Input: part model. Units: mm. Frame: model coordinates. Face numbers are marked on the shaded views. A direction names the side the tool comes from. Coordinates: 2 decimals unless noted, no trailing zeros. Loops run counter-clockwise (first coordinate to the right, second up) from the corner with the lowest first, then second, coordinate; pieces in that order, holes last. Notation, with made-up numbers: M 75,68 L 100,68 A28 cw 100,86 Z; hole C 30,-14 d11. An arc over 180 degrees is marked long. Use a Markdown table: item, result. Add a question column.
1. Section A-A on z = 0. Output: boundary loops of the cut face in (x, y), then the cut area to 3 significant figures.
2. Line query: L1, parallel to Y at x = 18, z = 18; L2, parallel to Y at x = 2.5, z = 13.5; L3, parallel to Z at x = 21, y = 36.5. Output: solid intervals per line, ascending. Write a range as [from, to].
3. Section C-C on x = 28. Output: boundary loops of the cut face in (y, z), then the cut area to 3 significant figures.
4. Pin query (flat end, axial travel): pin 1 (6 mm diameter, centred on x = 14.5, z = -2.5, fed in from +Y); pin 2 (3 mm diameter, centred on x = 17, z = 27.5, fed in from -Y); pin 3 (1.5 mm diameter, centred on x = 22, y = 1.5, fed in from -Z). Return the tip coordinate at first contact, or that it passes through.
5. Set-up query: the marked faces 1 and 2. Return all of +Z, -Z, +X, -X, +Y, -Y with unobstructed straight access to the full face (end or side cutting, diameter ignored); none if empty.
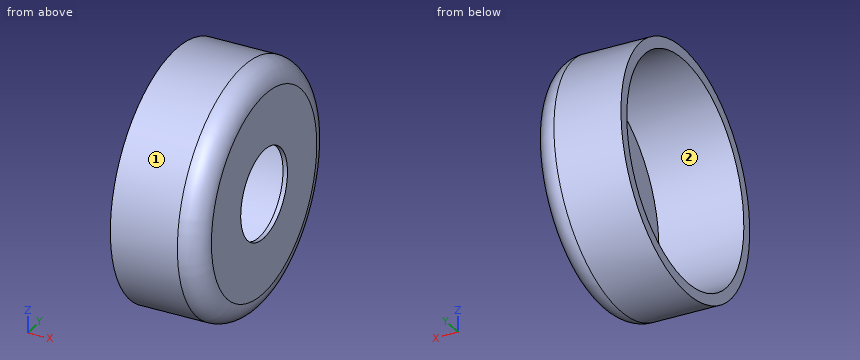
```python
from build123d import *

# Parameters (mm, degrees)
SKETCH1_R           = 55
BOSS_EXTRUDE1_DEPTH = 40
SKETCH2_R           = 50
CUT_EXTRUDE1_DEPTH  = 38
SKETCH3_R           = 20
CUT_EXTRUDE2_DEPTH  = 38
FILLET1_R           = 10


with BuildPart() as part:
    # Sketch1 → Boss-Extrude1 (new body)
    with BuildSketch(Plane(origin=(0, 0, 0), x_dir=(0, 0, -1), z_dir=(1, 0, 0))):
        Circle(SKETCH1_R)
    extrude(amount=BOSS_EXTRUDE1_DEPTH)

    # Sketch2 → Cut-Extrude1 (cut)
    with BuildSketch(Plane.ZY):
        Circle(SKETCH2_R)
    extrude(amount=-CUT_EXTRUDE1_DEPTH, mode=Mode.SUBTRACT)

    # Sketch3 → Cut-Extrude2 (cut)
    with BuildSketch(Plane(origin=(40, 0, 0), x_dir=(0, 0, -1), z_dir=(1, 0, 0))):
        Circle(SKETCH3_R)
    extrude(amount=-CUT_EXTRUDE2_DEPTH, mode=Mode.SUBTRACT)

    # Fillet1
    fillet1_edges = [part.edges().sort_by_distance(p)[0] for p in [
        (40, 0, 55),
    ]]
    fillet(fillet1_edges, radius=FILLET1_R)


solid = part.part
```
Answers below:
| question | item | result |
|---|---|---|
| 1 | outline | M 0,-55 L 30,-55 A10 ccw 40,-45 L 40,-20 L 38,-20 L 38,-50 L 0,-50 Z; M 0,50 L 38,50 L 38,20 L 40,20 L 40,45 A10 ccw 30,55 L 0,55 Z |
| 1 | area | 477 mm² |
| 2 | L1 | y = [-51.97, -46.65], [46.65, 51.97] |
| 2 | L2 | y = [-53.32, -48.14], [48.14, 53.32] |
| 2 | L3 | z = [-41.14, -34.17], [34.17, 41.14] |
| 3 | outline | C 0,0 d110; hole C 0,0 d100 |
| 3 | area | 1,650 mm² |
| 4 | pin 1 | stops at y = 55 |
| 4 | pin 2 | stops at y = -48.47 |
| 4 | pin 3 | stops at z = -54.99 |
| 5 | face 1 | +X, -X |
| 5 | face 2 | -X |
